```python
from build123d import *

# Parameters (mm, degrees)
CHAMFER_1_SIZE            = 3
CHAMFER_2_SIZE            = 2
CHAMFER_3_SIZE            = 1
SKETCH_2_R                = 2.5
CUT_EXTRUDE_1_DEPTH       = 50
HOLE_WIZARD_8_0_8_1_D     = 8
HOLE_WIZARD_8_0_8_1_DEPTH = 90
HOLE_WIZARD_8_0_8_1_TIP   = 2.403442476
HOLE_WIZARD_M14_1_D       = 12
HOLE_WIZARD_M14_1_DEPTH   = 45
HOLE_WIZARD_M14_1_TIP     = 3.605163714


with BuildPart() as part:
    # 草图1 → 旋转1 (revolve)
    with BuildSketch(Plane.XY, mode=Mode.PRIVATE) as revolve_1_sk:
        with BuildLine():
            Line((0, 0), (0, 30))
            Line((0, 30), (-11, 30))
            Line((-11, 30), (-11, 35))
            Line((-11, 35), (-80.641101056, 35))
            ThreePointArc((-80.641101056, 35), (-85, 34), (-89.358898944, 35))
            Line((-89.358898944, 35), (-224, 35))
            Line((-224, 35), (-224, 0))
            Line((-224, 0), (0, 0))
        make_face()
    revolve(revolve_1_sk.sketch.rotate(Axis((0, 0, 0), (-1, 0, 0)), 90), axis=Axis((0, 0, 0), (-1, 0, 0)))

    # 倒角1
    chamfer_1_edges = [part.edges().sort_by_distance(p)[0] for p in [
        (-224, 0, 35),
    ]]
    chamfer(chamfer_1_edges, length=CHAMFER_1_SIZE)

    # 倒角2
    chamfer_2_edges = [part.edges().sort_by_distance(p)[0] for p in [
        (0, 0, 30),
    ]]
    chamfer(chamfer_2_edges, length=CHAMFER_2_SIZE)

    # 倒角3
    chamfer_3_edges = [part.edges().sort_by_distance(p)[0] for p in [
        (-11, 0, 35),
    ]]
    chamfer(chamfer_3_edges, length=CHAMFER_3_SIZE)

    # 草图2 → 切除-拉伸1 (cut, symmetric)
    with BuildSketch(Plane(origin=(0, 0, 0), x_dir=(1, 0, 0), z_dir=(0, 1, 0))):
        with Locations(Location((-85, 0, 0), (0, 0, 134.50396252))):
            Circle(SKETCH_2_R)
    extrude(amount=CUT_EXTRUDE_1_DEPTH, both=True, mode=Mode.SUBTRACT)

    # Ø8.0 (8) 直径孔1
    with Locations(Plane(origin=(0, 0, 0), x_dir=(0, 0, 1), z_dir=(1, 0, 0))):
        with Locations((0, 0)):
            Hole(HOLE_WIZARD_8_0_8_1_D / 2, depth=HOLE_WIZARD_8_0_8_1_DEPTH)
            with Locations((0, 0, -(HOLE_WIZARD_8_0_8_1_DEPTH + HOLE_WIZARD_8_0_8_1_TIP / 2))):  # 118° drill point
                Cone(0, HOLE_WIZARD_8_0_8_1_D / 2, HOLE_WIZARD_8_0_8_1_TIP, mode=Mode.SUBTRACT)

    # M14 螺纹孔1
    with Locations(Plane(origin=(0, 0, 0), x_dir=(0, 0, 1), z_dir=(1, 0, 0))):
        with Locations((0, 0)):
            Hole(HOLE_WIZARD_M14_1_D / 2, depth=HOLE_WIZARD_M14_1_DEPTH)
            with Locations((0, 0, -(HOLE_WIZARD_M14_1_DEPTH + HOLE_WIZARD_M14_1_TIP / 2))):  # 118° drill point
                Cone(0, HOLE_WIZARD_M14_1_D / 2, HOLE_WIZARD_M14_1_TIP, mode=Mode.SUBTRACT)


solid = part.part
```
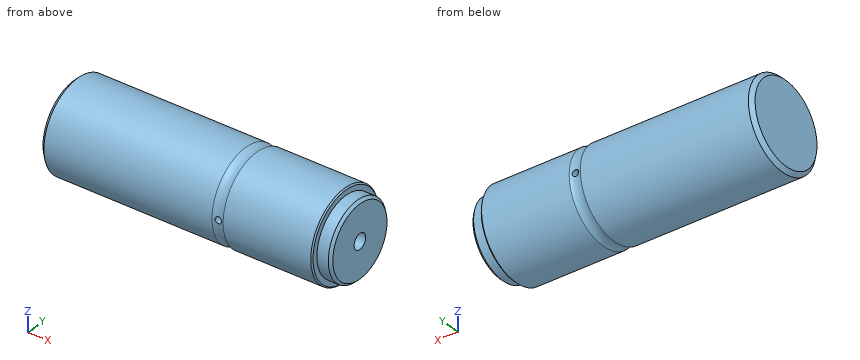
Geometry check sheet. Reference: the model listing, model coordinates, mm. Give positions to 0.01 mm unless a question says otherwise; leave off trailing zeros. Order: outer loops, then holes, each group sorted by start corner. A loop starts at its lowest first (then second) coordinate and runs counter-clockwise, first axis right, second up.
1. Section check B-B, the plane x = -112.5. Enter the section's corners in (y, z), and give its area (3 significant figures).
2. Gauge pin test, flat ends, axial feed: pin 1 Ø4 at (x, y) = (-41.5, 23.5) entering from +Z; pin 2 Ø4.5 at (x, z) = (-85, 0) entering from -Y; pin 3 Ø2 at (x, y) = (-84, 4) entering from -Z; pin 4 Ø13 at (y, z) = (0, 0) entering from +X. Record the tip position at first contact, or that the pin passes through.
3. Section check A-A, the plane x = -51. Enter the section's corners in (y, z).
4. Thickness scan on L1, parallel to X at y = -8.5, z = 0; L2, parallel to Y at x = -24, z = 0; L3, parallel to Y at x = -79, z = 0. Record the ranges inside material, lowest first.
Values follow:
1. outline: circle Ø70 at (0, 0)
1. area: 3,850 mm2
2. pin 1: stops at z = 27.62
2. pin 2: passes through
2. pin 3: stops at z = -34
2. pin 4: stops at x = 0
3. outline: circle Ø70 at (0, 0); hole circle Ø8 at (0, 0)
4. L1: x = -224 to -87.5, -82.5 to 0
4. L2: y = -35 to -6, 6 to 35
4. L3: y = -35 to -4, 4 to 35
